Design review of the part built by this model. Coordinates are the model's own, in mm. A direction names the side the tool comes from. Round coordinates to 2 decimals unless told otherwise and drop trailing zeros. Write each loop counter-clockwise with the first axis right and the second up, starting at its lowest first coordinate (ties: lowest second). Pieces come first, ordered by that corner, then holes. Notation, with made-up numbers: (13, -25) -> (63, -25) arc R29 ccw to (63, 5) -> close; hole circle Ø9 at (27.25, 76). An arc over 180 degrees is marked (long way). Write item = value, one per line. Start each with the question number.
Item 1: Mouldability with a two-part tool opening along Z and no side actions: class faces 1 (the flat face through (1, 10, 31)), 2 (the flat face through (65, 6, 0)), 3 (the flat face through (62, 14, 10)), 4 (the flat face through (1, 13, 24)) as released by +Z, released by -Z, zero draft, split by the parting line, or undercut.
Item 2: Add section A-A, the plane z = 5. State the section outline as (x, y) points, then the cut area to 3 significant figures.
Item 3: To check wall thickness, follow L1, parallel to Z at x = -61, y = 18.85; L2, parallel to Z at x = -17.5, y = 10.25; L3, parallel to X at y = 18, z = -27. State the ranges of each line that lie inside material, in increasing order.
Item 4: For pin 1 Ø5.5 at (x, z) = (-39, 17.5) entering from +Y; pin 2 Ø1.5 at (y, z) = (12, 5) entering from +X; pin 3 Ø1.5 at (x, z) = (-61, -27) entering from +Y, all flat-tipped, find the tip position at first contact; note any pin that passes through.
Item 5: Add section C-C, the plane y = 9.75. State the section outline as (x, z) points.
Item 6: Machinability: for faces 5 (the flat face through (-65, 10, 0)), 6 (the flat face through (62, 13, -10)), 7 (the flat face through (-1, 13, -24)), which of the approach directions +Z, -Z, +X, -X, +Y, -Y give a long, thin tool a straight path to every point of the face, cutting with its end or side? Answer none if there is none.
Item 7: Add section B-B, the plane x = -30.5. State the section outline as (y, z) points, then the cut area to 3 significant figures.
Solid Edge part; units mm, degrees
sketch "Sketch1" plane through (0, 0, 0) normal (0, -1, 0) x (1, 0, 0)
  line L0 (-65, -31) -> (65, -31)
  line L1 (65, -31) -> (65, 31)
  line L2 (65, 31) -> (-65, 31)
  line L3 (-65, 31) -> (-65, -31)
extrude "Ajout_matière_1" add sketch "Sketch1" against normal blind 20
shell "Coque_1" thickness 7 removed faces 1 at (-42.0333, 20, 21.2867)
fillet "Congé_1" radius 1 8 edges at (0, 0, -31) (65, 0, 0) (65, 10, -31) (-65, 10, -31) (-65, 0, 0) (-65, 10, 31) (0, 0, 31) (65, 10, 31)
sketch "Sketch2" plane through (65, 13, 0) normal (1, 0, 0) x (0, 0, -1)
  line L0 (-10, -6) -> (10, -6)
  line L1 (10, -6) -> (10, 7)
  line L2 (10, 7) -> (-10, 7)
  line L3 (-10, 7) -> (-10, -6)
extrude "Cutout1" cut sketch "Sketch2" against normal up to vertex (18.3022 mm away)
sketch "Sketch3" plane through (3.5, 7, 0) normal (0, 1, 0) x (0, 0, -1)
  line L0 (24, -40.5) -> (11, -40.5)
  line L1 (11, -40.5) -> (11, -54.5)
  line L2 (11, -54.5) -> (24, -54.5)
  line L3 (24, -54.5) -> (24, -40.5)
  line L4 (-24, 45.5) -> (-14, 45.5)
  line L5 (-14, 45.5) -> (-14, 38.5)
  line L6 (-14, 38.5) -> (-24, 38.5)
  line L7 (-24, 38.5) -> (-24, 45.5)
  line L8 (24, -21.5) -> (8, -21.5)
  line L9 (8, -21.5) -> (8, -28.5)
  line L10 (8, -28.5) -> (24, -28.5)
  line L11 (24, -28.5) -> (24, -21.5)
  line L12 (-24, -45.5) -> (-14, -45.5)
  line L13 (-14, -45.5) -> (-14, -36.5)
  line L14 (-14, -36.5) -> (-24, -36.5)
  line L15 (-24, -36.5) -> (-24, -45.5)
  dimension "D1" = 14
  dimension "D2" = 14
  dimension "D3" = 14
  dimension "D4" = 24
  dimension "D5" = 24
  dimension "D6" = 11
  dimension "D7" = 8
  dimension "D8" = 24
extrude "Ajout_matière_2" add sketch "Sketch3" along normal blind 1
hole "Perçage_1" at (61, 20, -27) direction (0, -1, 0) diameter 1.713 depth 5 thread major 2.2 thread length 2
hole "Hole1" at (61, 20, 27) direction (0, -1, 0) diameter 1.713 depth 5 thread major 2.2 thread length 2
hole "Hole2" at (-61, 20, -27) direction (0, -1, 0) diameter 1.713 depth 5 thread major 2.2 thread length 2
hole "Hole3" at (-61, 20, 27) direction (0, -1, 0) diameter 1.713 depth 5 thread major 2.2 thread length 2
hole "Perçage_5" at (-38.3344, 8, 16.7401) direction (0, -1, 0) diameter 1.713 depth 5
hole "Hole4" at (28.6915, 8, -9.7518) direction (0, -1, 0) diameter 1.713 depth 5
hole "Hole5" at (47.6833, 8, -13.2632) direction (0, -1, 0) diameter 1.713 depth 5
hole "Hole6" at (44.6933, 8, 16.7289) direction (0, -1, 0) diameter 1.713 depth 5
properties material "Pin"
Result set:
q1.face_1 = released by +Z
q1.face_2 = zero draft
q1.face_3 = undercut
q1.face_4 = undercut
q2.outline = (-65, 1) arc R1 ccw to (-64, 0) -> (64, 0) arc R1 ccw to (65, 1) -> (65, 7) -> (-58, 7) -> (-58, 20) -> (-65, 20) -> close
q2.area = 1,000 mm²
q3.L1 = -31 to -27.86, -26.14 to 26.14, 27.86 to 31
q3.L2 = -31 to -24, 24 to 31
q3.L3 = -65 to -61.86, -60.14 to 60.14, 61.86 to 65
q4.pin_1 = 8
q4.pin_2 = -58
q4.pin_3 = 15
q5.outline = (-65, -30) arc R1 ccw to (-64, -31) -> (64, -31) arc R1 ccw to (65, -30) -> (65, -10) -> (58, -10) -> (58, -24) -> (-58, -24) -> (-58, 24) -> (58, 24) -> (58, 10) -> (65, 10) -> (65, 30) arc R1 ccw to (64, 31) -> (-64, 31) arc R1 ccw to (-65, 30) -> close
q6.face_5 = +Z, -Z, -X, +Y, -Y
q6.face_6 = +X, +Y
q6.face_7 = +Y
q7.outline = (0, -30) arc R1 ccw to (1, -31) -> (20, -31) -> (20, -24) -> (7, -24) -> (7, 24) -> (20, 24) -> (20, 31) -> (1, 31) arc R1 ccw to (0, 30) -> close
q7.area = 616 mm²
